Can you work these out from the model? Positions are in its coordinate system, mm. A direction names the side the tool comes from. Coordinates: 2 decimals unless noted, no trailing zeros. Order: outer loops, then holes, each group sorted by start corner. A loop starts at its lowest first (then second) coordinate and runs counter-clockwise, first axis right, second up. Notation, with made-up numbers: M -24.75,8.5 L 0.25,8.5 A22 ccw 0.25,20.5 Z; hole C 58,-30.5 d2. An arc over 180 degrees is marked long. Answer as a JSON object with one key per item and string values.
from build123d import *

# Parameters (mm, degrees)
F3_DEPTH = 92.038
F4_W     = 44.9782982225
F4_H     = 128.527504392
F5_DEPTH = 25
F7_DEPTH = 50


with BuildPart() as f3:
    # F2 (on line) → F3 (new body)
    with BuildSketch(Plane(origin=(0, 0, 0), x_dir=(0.9659258263, 0, 0.2588190451), z_dir=(0.2588190451, 0, -0.9659258263))):
        with BuildLine():
            Line((-10.2108, -12.7), (10.2108, -12.7))
            ThreePointArc((10.2108, -12.7), (11.9709301997, -11.9709301997), (12.7, -10.2108))
            Line((12.7, -10.2108), (12.7, 10.2108))
            ThreePointArc((12.7, 10.2108), (11.9709301997, 11.9709301997), (10.2108, 12.7))
            Line((10.2108, 12.7), (-10.2108, 12.7))
            ThreePointArc((-10.2108, 12.7), (-11.9709301997, 11.9709301997), (-12.7, 10.2108))
            Line((-12.7, 10.2108), (-12.7, -10.2108))
            ThreePointArc((-12.7, -10.2108), (-11.9709301997, -11.9709301997), (-10.2108, -12.7))
        make_face()
        with BuildLine():
            ThreePointArc((11.4554, -10.2108), (11.0908650999, -11.0908650999), (10.2108, -11.4554))
            Line((10.2108, -11.4554), (-10.2108, -11.4554))
            ThreePointArc((-10.2108, -11.4554), (-11.0908650999, -11.0908650999), (-11.4554, -10.2108))
            Line((-11.4554, -10.2108), (-11.4554, 10.2108))
            ThreePointArc((-11.4554, 10.2108), (-11.0908650999, 11.0908650999), (-10.2108, 11.4554))
            Line((-10.2108, 11.4554), (10.2108, 11.4554))
            ThreePointArc((10.2108, 11.4554), (11.0908650999, 11.0908650999), (11.4554, 10.2108))
            Line((11.4554, 10.2108), (11.4554, -10.2108))
        make_face(mode=Mode.SUBTRACT)
    extrude(amount=F3_DEPTH)

    # F4 (on Front) → F5 (cut, symmetric)
    with BuildSketch(Plane.XZ):
        with Locations((-10.2218911174, -60.9767503232)):
            Rectangle(F4_W, F4_H)
    extrude(amount=F5_DEPTH, both=True, mode=Mode.SUBTRACT)

    # F6 (on Right) → F7 (cut)
    with BuildSketch(Plane.YZ):
        with BuildLine():
            Line((0, -155.816540122), (55.8327542288, -89.3573068549))
            ThreePointArc((55.8327542288, -89.3573068549), (2.0772321925, -84.2070783197), (-51.7434931467, -88.6241505764))
            Line((-51.7434931467, -88.6241505764), (0, -155.816540122))
        make_face()
    extrude(amount=F7_DEPTH, mode=Mode.SUBTRACT)


solid = f3.part
Item 1: Please list where these lines run through material, in increasing order: line 1 (Y direction, x = 23.5, z = -72.5); line 2 (X direction, y = 11, z = -62); line 3 (X direction, y = 2.5, z = -61).
Answers follow:
{"line 1": "y = -12.7 to -11.46, 11.46 to 12.7", "line 2": "x = 28.18 to 29.63", "line 3": "x = 28.2 to 29.49"}
Item 2: Which directions (+Z, -Z, +X, -X, +Y, -Y) give clear straight access to the entire face, cutting with the end or side of a thin tool? Please do faces 4 (the flat face through (17, 11.455, -55)), 5 (the cylindrical face through (23.162, -11.951, -40.116)).
Answers follow:
{"face 4": "-Z, -X", "face 5": "+Z, +X, -Y"}
Item 3: I want a section at A-A, the plane y = -0.5. Write out the boundary of the cut face in (x, z).
Answers follow:
{"outline": "M 12.27,-1.52 L 34.42,-84.2 L 35.71,-84.2 L 12.27,3.29 Z"}
Item 4: I want a section at B-B, the plane y = 6.5. Write out the boundary of the cut face in (x, z), plus the area to 3 significant figures.
Answers follow:
{"outline": "M 12.27,-1.52 L 34.44,-84.27 L 35.73,-84.27 L 12.27,3.29 Z", "area": "110 mm^2"}
Item 5: I'm going to push flat-ended pins straight in: pin 1 (12 mm diameter, centred on x = 33, z = -55.5, fed in from -Y); pin 2 (1.5 mm diameter, centred on x = 22.5, z = -34.5, fed in from +Y); pin 3 (4 mm diameter, centred on y = -3.5, z = -49, fed in from +X). Where does each tip first touch, or does it pass through?
Answers follow:
{"pin 1": "stops at y = -12.33", "pin 2": "stops at y = 11.88", "pin 3": "stops at x = 26.81"}
Item 6: If we mould it in two halves opening along Y, with no side actions, what happens to faces 1 (the cylindrical face through (22.85, -11.1, -42.47)), 2 (the flat face through (20, 12.7, -64)), 3 (the flat face through (12.267, 12, -28))? For each: pulls with the +Y half, pulls with the -Y half, needs draft (parallel to the pull), parting line crosses it, or undercut.
Answers follow:
{"face 1": "undercut", "face 2": "pulls with the +Y half", "face 3": "needs draft"}
